The model under review builds one solid part; all positions refer to its coordinate system, in mm. A direction names the side the tool comes from. Give positions to 0.01 mm unless a question says otherwise; leave off trailing zeros. Order: outer loops, then holes, each group sorted by start corner. A loop starts at its lowest first (then second) coordinate and runs counter-clockwise, first axis right, second up.
```python
from build123d import *

# Parameters (mm, degrees)
SALIENTE_EXTRUIR1_DEPTH = 150
CROQUIS4_W              = 20
CROQUIS4_H              = 40
CORTAR_EXTRUIR1_DEPTH   = 30
CROQUIS5_R              = 5
CORTAR_EXTRUIR2_DEPTH   = 52


with BuildPart() as part:
    # Croquis1 → Saliente-Extruir1 (new body)
    with BuildSketch(Plane.XY):
        with BuildLine():
            Line((-22.5, -20), (22.5, -20))
            ThreePointArc((22.5, -20), (42.5, 0), (22.5, 20))
            Line((22.5, 20), (-22.5, 20))
            Line((-22.5, 20), (-22.5, -20))
        make_face()
    extrude(amount=SALIENTE_EXTRUIR1_DEPTH)

    # Croquis4 → Cortar-Extruir1 (cut)
    with BuildSketch(Plane.XY.offset(150)):
        with Locations((32.5, 0)):
            Rectangle(CROQUIS4_W, CROQUIS4_H)
    extrude(amount=-CORTAR_EXTRUIR1_DEPTH, mode=Mode.SUBTRACT)

    # Croquis5 → Cortar-Extruir2 (cut)
    with BuildSketch(Plane.ZY.offset(22.5)):
        with Locations((135, 0)):
            Circle(CROQUIS5_R)
    extrude(amount=-CORTAR_EXTRUIR2_DEPTH, mode=Mode.SUBTRACT)


solid = part.part
```
1. Draft analysis for pull direction X (two halves, no side actions). For faces 3 (the flat face through (0, 20, 74)), 4 (the flat face through (22.5, -5, 132)), 5 (the flat face through (-22.5, 0, 74)), state which applies: pulls with the +X half, pulls with the -X half, needs draft (parallel to the pull), parting line crosses it, or undercut.
2. Take a section at A-A (y = 0). Write out the cut boundary in (x, z), and give its area (3 significant figures).
3. Take a section at B-B (z = 135). Write out the cut boundary in (x, y), and give its area (3 significant figures).
4. Insertion check: pin 1 (6 mm diameter, centred on y = -9, z = 90.5, fed in from +X); pin 2 (1.5 mm diameter, centred on x = 31, y = -9, fed in from +Z); pin 3 (1.5 mm diameter, centred on y = 9, z = 77.5, fed in from +X). Each pin has a flat end and moves straight along its axis. Give the tip position at first contact, or say it passes through.
5. For faces 1 (the flat face through (30, 0, 120)), 2 (the cylindrical face through (-0.32, 1.5, 139.77)), list the 3-axis set-ups (+Z, -Z, +X, -X, +Y, -Y) from which the entire face can be reached by the end or side of a thin tool; tool diameter is ignored.
6. Take a section at C-C (z = 27.5). Write out the cut boundary in (x, y).
7. Take a section at D-D (y = 12.5). Write out the cut boundary in (x, z).
8. To check wall thickness, follow line 1 (Y direction, x = -10.5, z = 135); line 2 (Z direction, x = 23.5, y = 3); line 3 (X direction, y = -13, z = 36.5). State the ranges of each line that lie inside material, in increasing order.
Answer:
1. face 3: needs draft
1. face 4: pulls with the +X half
1. face 5: pulls with the -X half
2. outline: (-22.5, 0) - (42.5, 0) - (42.5, 120) - (22.5, 120) - (22.5, 130) - (-22.5, 130) - close; (-22.5, 140) - (22.5, 140) - (22.5, 150) - (-22.5, 150) - close
2. area: 8,700 mm2
3. outline: (-22.5, -20) - (22.5, -20) - (22.5, -5) - (-22.5, -5) - close; (-22.5, 5) - (22.5, 5) - (22.5, 20) - (-22.5, 20) - close
3. area: 1,350 mm2
4. pin 1: stops at x = 41.58
4. pin 2: stops at z = 120
4. pin 3: stops at x = 40.72
5. face 1: +Z, +X, +Y, -Y
5. face 2: +X, -X
6. outline: (-22.5, -20) - (22.5, -20) arc R20 ccw to (22.5, 20) - (-22.5, 20) - close
7. outline: (-22.5, 0) - (38.11, 0) - (38.11, 120) - (22.5, 120) - (22.5, 150) - (-22.5, 150) - close
8. line 1: y = -20 to -5, 5 to 20
8. line 2: z = 0 to 120
8. line 3: x = -22.5 to 37.7
